Can you work these out from the drawing? Everything is in mm from the part's minimum corner. A direction names the side the tool comes from. Coordinates: 2 decimals unless noted, no trailing zeros. Loops run counter-clockwise (first coordinate to the right, second up) from the corner with the lowest first, then second, coordinate; pieces in that order, holes last. Notation, with made-up numbers: M 69.25,-13 L 121.25,-13 A29 cw 121.25,18 Z; hole C 34,1 d11. An arc over 180 degrees is marked long. Write each question's results on one line, items separated by ' | '.
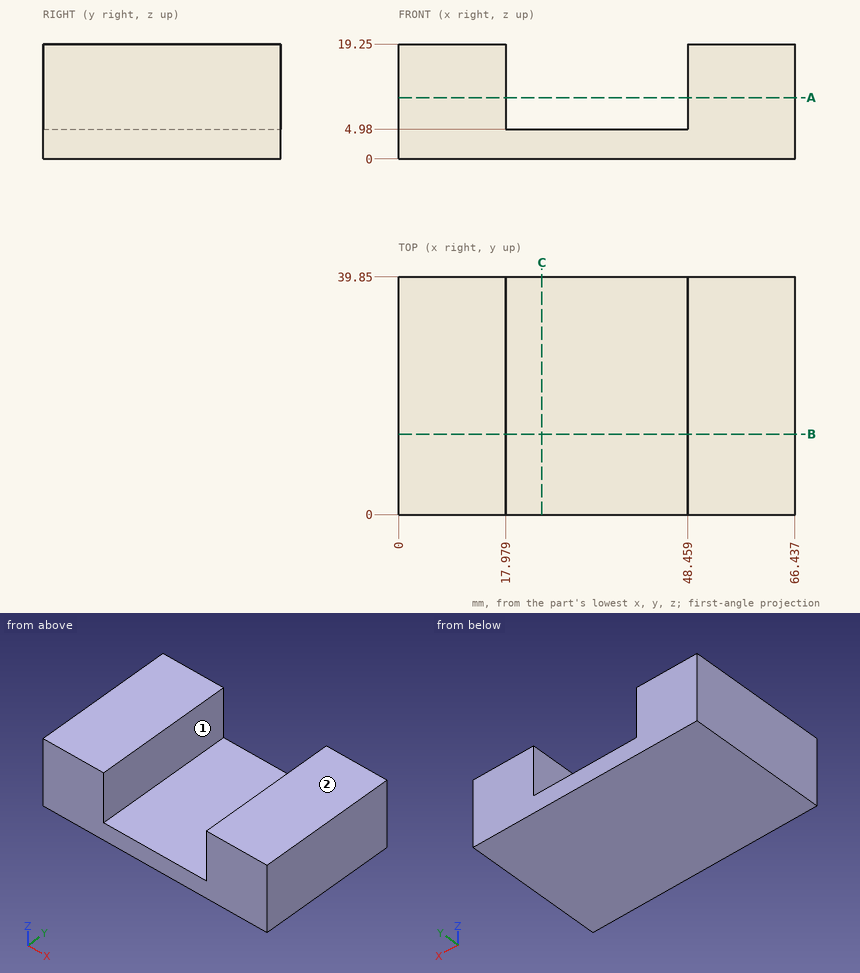
(1) Will these pins go through, and if not, where does the flat tip stop? P1, Ø12, axis at x = 44.5, y = 16, coming from the +Z side; P2, Ø12, axis at x = 39.5, y = 29, coming from the +Z side.
Reported:
P1: stops at z = 19.25 | P2: stops at z = 4.98
(2) Please list where these lines run through material, in increasing order: probe 1 along X at (y, z) = (11, 12.5); probe 2 along Z at (x, y) = (23.5, 30.5). Write a range as from..to.
Reported:
probe 1: x = 0..17.98, 48.46..66.44 | probe 2: z = 0..4.98
(3) Imagine slicing it at C-C, the plane x = 24. List the corners of the cut face in (y, z) for me.
Reported:
outline: M 0,0 L 39.85,0 L 39.85,4.98 L 0,4.98 Z
(4) Imagine slicing it at B-B, the plane y = 13.5. List the corners of the cut face in (x, z) for me.
Reported:
outline: M 0,0 L 66.44,0 L 66.44,19.25 L 48.46,19.25 L 48.46,4.98 L 17.98,4.98 L 17.98,19.25 L 0,19.25 Z
(5) Imagine slicing it at A-A, the plane z = 10.25. List the corners of the cut face in (x, y) for me, and give its area (3 significant figures).
Reported:
outline: M 0,0 L 17.98,0 L 17.98,39.85 L 0,39.85 Z; M 48.46,0 L 66.44,0 L 66.44,39.85 L 48.46,39.85 Z | area: 1,430 mm2
(6) Which directions (+Z, -Z, +X, -X, +Y, -Y) give clear straight access to the entire face, cutting with the end or side of a thin tool? Please do the marked faces 1 and 2.
Reported:
face 1: +Z, +Y, -Y | face 2: +Z, +X, -X, +Y, -Y
